For this review, take the finished solid that the model builds, in its own axes (mm). A direction names the side the tool comes from. Give positions to 0.01 mm unless a question says otherwise; leave off trailing zeros. Loops run counter-clockwise (first coordinate to the right, second up) from the corner with the lowest first, then second, coordinate; pieces in that order, holes last. Notation, with made-up numbers: (52.5, -38.5) -> (92.5, -38.5) arc R21 ccw to (92.5, -21.5) -> close; hole circle Ø10 at (-30.5, 78.25). An arc over 180 degrees is marked (long way). Write each question's results on one line, items separated by ' | '. Start each with the question number.
```python
from build123d import *

# Parameters (mm, degrees)
SKETCH1_W               = 143
SKETCH1_H               = 52
SKETCH1_R               = 1.6
BOSS_EXTRUDE1_DEPTH     = 3
CUT_EXTRUDE1_DEPTH      = 77.139674284
CUT_EXTRUDE1_DEPTH_BACK = 10
SKETCH2_W               = 26
SKETCH2_H               = 6
SKETCH2_W_2             = 22
SKETCH2_W_3             = 27
SKETCH2_W_4             = 9
SKETCH2_H_2             = 18
SKETCH4_W               = 50
SKETCH4_H               = 5
SKETCH4_W_2             = 37
CUT_EXTRUDE2_DEPTH      = 3
SKETCH5_R               = 2.05
SKETCH5_R_2             = 19
CUT_EXTRUDE3_DEPTH      = 3
CUT_EXTRUDE4_DEPTH      = 3


with BuildPart() as part:
    # Sketch1 → Boss-Extrude1 (new body)
    with BuildSketch(Plane.XY):
        Rectangle(SKETCH1_W, SKETCH1_H)
        with Locations((-67.75, 21.75)):
            Circle(SKETCH1_R, mode=Mode.SUBTRACT)
        with Locations((-67.75, -21.75)):
            Circle(SKETCH1_R, mode=Mode.SUBTRACT)
        with Locations((67.75, 21.75)):
            Circle(SKETCH1_R, mode=Mode.SUBTRACT)
        with Locations((67.75, -21.75)):
            Circle(SKETCH1_R, mode=Mode.SUBTRACT)
    extrude(amount=BOSS_EXTRUDE1_DEPTH)

    # Sketch2 → Cut-Extrude1 (cut, two sides: drawn at the far end of the back side and taken through both)
    with BuildSketch(Plane.XY.offset(3).offset(-CUT_EXTRUDE1_DEPTH_BACK)):
        with Locations((-34.75, -23)):
            Rectangle(SKETCH2_W, SKETCH2_H)
        with Locations((2.25, -23)):
            Rectangle(SKETCH2_W_2, SKETCH2_H)
        with Locations((43.75, -23)):
            Rectangle(SKETCH2_W_3, SKETCH2_H)
        with Locations((-67, -6.75)):
            Rectangle(SKETCH2_W_4, SKETCH2_H_2)
    extrude(amount=CUT_EXTRUDE1_DEPTH + CUT_EXTRUDE1_DEPTH_BACK, mode=Mode.SUBTRACT)

    # Sketch4 → Cut-Extrude2 (cut)
    with BuildSketch(Plane.XY.offset(3)):
        with Locations((-29.75, 23.5)):
            Rectangle(SKETCH4_W, SKETCH4_H)
        with Locations((36.75, 23.5)):
            Rectangle(SKETCH4_W_2, SKETCH4_H)
    extrude(amount=-CUT_EXTRUDE2_DEPTH, mode=Mode.SUBTRACT)

    # Sketch5 → Cut-Extrude3 (cut)
    with BuildSketch(Plane.XY.offset(3)):
        with Locations((52, -15)):
            Circle(SKETCH5_R)
        with Locations((20, -15)):
            Circle(SKETCH5_R)
        with Locations((20, 17)):
            Circle(SKETCH5_R)
        with Locations((52, 17)):
            Circle(SKETCH5_R)
        with Locations((36, 1)):
            Circle(SKETCH5_R_2)
    cut_extrude3 = extrude(amount=-CUT_EXTRUDE3_DEPTH, mode=Mode.SUBTRACT)

    # Mirror1: Cut-Extrude3 across plane
    add(cut_extrude3.mirror(Plane(origin=(0, 0, 0), x_dir=(0, 0, 1), z_dir=(1, 0, 0))), mode=Mode.SUBTRACT)

    # Sketch6 → Cut-Extrude4 (cut)
    with BuildSketch(Plane.XY.offset(3)):
        with BuildLine():
            Line((6, -5), (6, 5))
            ThreePointArc((6, 5), (9, 8), (12, 5))
            Line((12, 5), (12, -5))
            ThreePointArc((12, -5), (9, -8), (6, -5))
        make_face()
        with BuildLine():
            Line((-6, -5), (-6, 5))
            ThreePointArc((-6, 5), (-9, 8), (-12, 5))
            Line((-12, 5), (-12, -5))
            ThreePointArc((-12, -5), (-9, -8), (-6, -5))
        make_face()
    extrude(amount=-CUT_EXTRUDE4_DEPTH, mode=Mode.SUBTRACT)


solid = part.part
```
1. Machinability: for faces 4 (the flat face through (-47.75, -23, 1)), 5 (the flat face through (-67, 2.25, 1)), 6 (the flat face through (-54.75, 23, 2)), 7 (the cylindrical face through (9, 8, 2)), which of the approach directions +Z, -Z, +X, -X, +Y, -Y give a long, thin tool a straight path to every point of the face, cutting with its end or side? Answer none if there is none.
2. Draft analysis for pull direction Y (two halves, no side actions). For faces 1 (the flat face through (-4.75, 23, 2)), 2 (the flat face through (44, -20, 1)), 3 (the flat face through (-12, 0, 2)), state which applies: released by +Y, released by -Y, zero draft, split by the parting line, or undercut.
3. We need section D-D (z = 2). Count the separate pieces of the cut face and the enclosed holes in it, plus the area to 3 significant figures.
4. We need section B-B (x = -36). Write out the cut boundary in (y, z), plus the area to 3 significant figures.
5. We need section C-C (y = 13). Write out the cut boundary in (x, z).
6. We need section A-A (y = -21.75). Write out the cut boundary in (x, z), plus the area to 3 significant figures.
7. For pin 1 Ø1.5 at (x, y) = (-49, -16) entering from -Z; pin 2 Ø2.5 at (x, y) = (-20, 17) entering from +Z, all flat-tipped, find the tip position at first contact; note any pin that passes through.
8. Wall thickness on L1, parallel to Y at x = -67.75, z = 0.7; L2, parallel to Y at x = 52, z = 1.75; L3, parallel to X at y = -20.5, z = 0.4: over which ranges is each line inside the solid? List them lowest first.
Response:
1) face 4: +Z, -Z, -Y | face 5: +Z, -Z, -X | face 6: +Z, -Z, +Y | face 7: +Z, -Z
2) face 1: zero draft | face 2: released by -Y | face 3: undercut
3) separate pieces: 1 | enclosed holes: 16 | area: 3,810 mm2
4) outline: (-20, 0) -> (-18, 0) -> (-18, 3) -> (-20, 3) -> close; (20, 0) -> (21, 0) -> (21, 3) -> (20, 3) -> close | area: 9.00 mm2
5) outline: (-71.5, 0) -> (-50.73, 0) -> (-50.73, 3) -> (-71.5, 3) -> close; (-21.27, 0) -> (21.27, 0) -> (21.27, 3) -> (-21.27, 3) -> close; (50.73, 0) -> (71.5, 0) -> (71.5, 3) -> (50.73, 3) -> close
6) outline: (-71.5, 0) -> (-69.35, 0) -> (-69.35, 3) -> (-71.5, 3) -> close; (-66.15, 0) -> (-47.75, 0) -> (-47.75, 3) -> (-66.15, 3) -> close; (-21.75, 0) -> (-8.75, 0) -> (-8.75, 3) -> (-21.75, 3) -> close; (13.25, 0) -> (30.25, 0) -> (30.25, 3) -> (13.25, 3) -> close; (57.25, 0) -> (66.15, 0) -> (66.15, 3) -> (57.25, 3) -> close; (69.35, 0) -> (71.5, 0) -> (71.5, 3) -> (69.35, 3) -> close | area: 185 mm2
7) pin 1: stops at z = 0 | pin 2: passes through
8) L1: y = -26 to -23.35, -20.15 to -15.75, 2.25 to 20.15, 23.35 to 26 | L2: y = -20 to -17.05, -12.95 to -9.25, 11.25 to 14.95, 19.05 to 21 | L3: x = -71.5 to -68.75, -66.75 to -47.75, -21.75 to -8.75, 13.25 to 30.25, 57.25 to 66.75, 68.75 to 71.5
